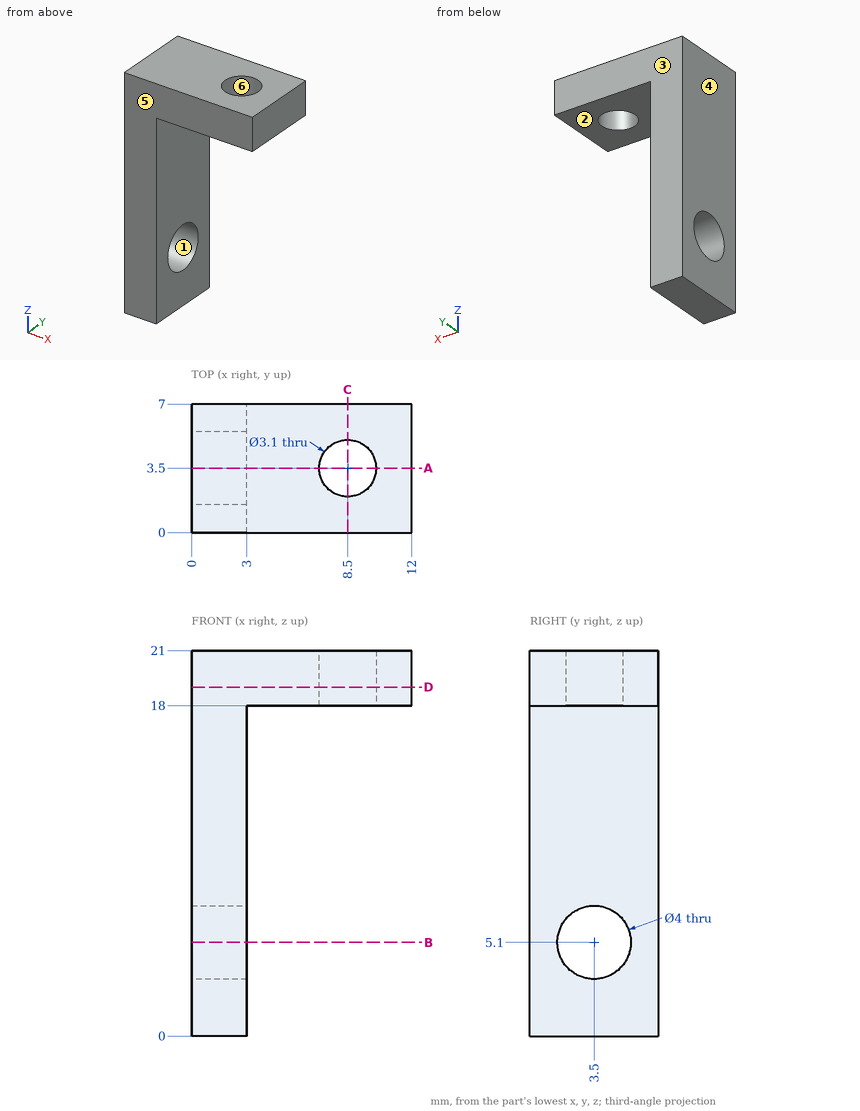
Drawing for the job (mm, zero at the part's lowest x, y, z). A direction names the side the tool comes from. Coordinates: 2 decimals unless noted, no trailing zeros. Order: outer loops, then holes, each group sorted by start corner. A loop starts at its lowest first (then second) coordinate and runs counter-clockwise, first axis right, second up. Notation, with made-up numbers: (-33, 89) -> (4, 89) arc R23 ccw to (4, 128) -> close; hole circle Ø11 at (-4.5, 31). An arc over 180 degrees is marked (long way). One line per item, written item: value.
(1) Mould opens along Y. For the marked faces 3, 4, 5 and 6 say: pulls with the +Y half, pulls with the -Y half, needs draft (parallel to the pull), parting line crosses it, or undercut.
Checked values:
face 3: pulls with the +Y half
face 4: needs draft
face 5: pulls with the -Y half
face 6: undercut
(2) Slice it at B-B, the plane z = 5.1. List the corners of the cut face in (x, y), plus the area to 3 significant figures.
Checked values:
outline: (0, 0) -> (3, 0) -> (3, 1.5) -> (0, 1.5) -> close; (0, 5.5) -> (3, 5.5) -> (3, 7) -> (0, 7) -> close
area: 9.00 mm2
(3) Slice it at A-A, the plane y = 3.5. List the corners of the cut face in (x, z).
Checked values:
outline: (0, 0) -> (3, 0) -> (3, 3.1) -> (0, 3.1) -> close; (0, 7.1) -> (3, 7.1) -> (3, 18) -> (6.95, 18) -> (6.95, 21) -> (0, 21) -> close; (10.05, 18) -> (12, 18) -> (12, 21) -> (10.05, 21) -> close
(4) Slice it at D-D, the plane z = 19. List the corners of the cut face in (x, y).
Checked values:
outline: (0, 0) -> (12, 0) -> (12, 7) -> (0, 7) -> close; hole circle Ø3.1 at (8.5, 3.5)
(5) Drop flat-ended pins along their axis: pin 1 Ø3 at (x, z) = (3, 16.5) entering from -Y; pin 2 Ø4 at (x, y) = (7.5, 3) entering from -Z. Give the stop position or say it passes through.
Checked values:
pin 1: y = 0
pin 2: z = 18
(6) Tool access for the marked faces 1 and 2: list every direction of +Z, -Z, +X, -X, +Y, -Y with a clear straight run to the whole face (end or side of a thin tool).
Checked values:
face 1: +X, -X
face 2: -Z, +X, +Y, -Y
(7) Probe line 1 (Z direction, x = 6, y = 1.5); line 2 (X direction, y = 5, z = 8); line 3 (Y direction, x = 2.25, z = 3.5). List the from-to ranges inside material, lowest first. Write a range as [from, to].
Checked values:
line 1: [18, 21]
line 2: [0, 3]
line 3: [0, 2.3], [4.7, 7]
(8) Slice it at C-C, the plane x = 8.5. List the corners of the cut face in (y, z).
Checked values:
outline: (0, 18) -> (1.95, 18) -> (1.95, 21) -> (0, 21) -> close; (5.05, 18) -> (7, 18) -> (7, 21) -> (5.05, 21) -> close
